The listing builds one solid part. Answer for the finished solid, in the listing's coordinates (mm). Face numbers are marked on the shaded views. A direction names the side the tool comes from. Round coordinates to 2 decimals unless told otherwise and drop trailing zeros. Order: outer loops, then holes, each group sorted by start corner. A loop starts at its lowest first (then second) coordinate and runs counter-clockwise, first axis right, second up. Notation, with made-up numbers: (-34.5, 68.5) -> (-0.5, 68.5) arc R19 ccw to (-0.5, 103.5) -> close; hole circle Ø9 at (38.5, 34). An arc over 180 degrees is marked (long way). Return JSON: item names as keys, results as strings. Group by question number.
(1) Determine the mould class of the marked faces 3, 4 and 5 for opening direction Z: +Z half, -Z half, draft (parallel to the pull), parting line (faces both ways), or undercut.
(2) The part is cut by section B-B (z = 0). Determine the outline of the cut face in (x, y), plus the area to 3 significant figures.
(3) Which of the six approach directions +Z, -Z, +X, -X, +Y, -Y give full straight-line access (tool end or side, diameter ignored) to the marked faces 1 and 2?
(4) The part is cut by section C-C (z = 5). Determine the outline of the cut face in (x, y), plus the area to 3 significant figures.
(5) The part is cut by section A-A (y = 0). Determine the outline of the cut face in (x, z).
(6) Each of these flat-tipped pins is pushed along its axis until it touches: pin 1 (12 mm diameter, centred on x = 34, y = 11.5, fed in from +Z); pin 2 (4.5 mm diameter, centred on x = 53, y = -4.5, fed in from +Z); pin 3 (5 mm diameter, centred on x = 73.5, z = 12.5, fed in from +Y). Where does it stop, or does it pass through?
(7) The part is cut by section D-D (y = -9.5). Determine the outline of the cut face in (x, z), plus the area to 3 significant figures.
(8) Consider line 1 (X direction, y = -4, z = 2.5); line 2 (Z direction, x = 28, y = -0.5); line 3 (Y direction, x = 83.5, z = -7.5). Determine where each line is inside the solid, lowest interval first. Write a range as [from, to].
from build123d import *

# Parameters (mm, degrees)
SKETCH1_R                           = 20
BOSS_EXTRUDE1_DEPTH                 = 105
CUT_EXTRUDE1_REACH                  = 110.743
CUT_EXTRUDE1_END_RADIUS             = 20
SKETCH2_W                           = 15
SKETCH2_H                           = 15
CUT_EXTRUDE1_DIRECTION_2_REACH      = 110.743
CUT_EXTRUDE1_DIRECTION_2_END_RADIUS = 20


with BuildPart() as part:
    # Sketch1 → Boss-Extrude1 (new body)
    with BuildSketch(Plane(origin=(0, 0, 0), x_dir=(0, 0, -1), z_dir=(1, 0, 0))):
        Circle(SKETCH1_R)
    extrude(amount=BOSS_EXTRUDE1_DEPTH)

    # Cut-Extrude1: up to this cylinder (the profile starts inside it)
    cut_extrude1_end = Plane(origin=(52.5, 0, 0), z_dir=(-1, 0, 0)) * Cylinder(CUT_EXTRUDE1_END_RADIUS, 262.486, mode=Mode.PRIVATE)
    # Sketch2 → Cut-Extrude1 (cut, up to the surface)
    with BuildSketch(Plane(origin=(0, 0, 0), x_dir=(1, 0, 0), z_dir=(0, 1, 0)), mode=Mode.PRIVATE) as cut_extrude1_sk1:
        with Locations((52.5, 0)):
            Rectangle(SKETCH2_W, SKETCH2_H)
    cut_extrude1_tool1 = extrude(cut_extrude1_sk1.sketch, amount=-CUT_EXTRUDE1_REACH, mode=Mode.PRIVATE) & cut_extrude1_end
    add(cut_extrude1_tool1.solids().sort_by_distance((52.5, 0, 0))[0], mode=Mode.SUBTRACT)

    # Cut-Extrude1 direction 2: up to this cylinder (the profile starts inside it)
    cut_extrude1_direction_2_end = Plane(origin=(52.5, 0, 0), z_dir=(-1, 0, 0)) * Cylinder(CUT_EXTRUDE1_DIRECTION_2_END_RADIUS, 262.486, mode=Mode.PRIVATE)
    # Sketch2 → Cut-Extrude1 direction 2 (cut, up to the surface)
    with BuildSketch(Plane(origin=(0, 0, 0), x_dir=(1, 0, 0), z_dir=(0, 1, 0)), mode=Mode.PRIVATE) as cut_extrude1_direction_2_sk1:
        with Locations((52.5, 0)):
            Rectangle(SKETCH2_W, SKETCH2_H)
    cut_extrude1_direction_2_tool1 = extrude(cut_extrude1_direction_2_sk1.sketch, amount=CUT_EXTRUDE1_DIRECTION_2_REACH, mode=Mode.PRIVATE) & cut_extrude1_direction_2_end
    add(cut_extrude1_direction_2_tool1.solids().sort_by_distance((52.5, 0, 0))[0], mode=Mode.SUBTRACT)


solid = part.part
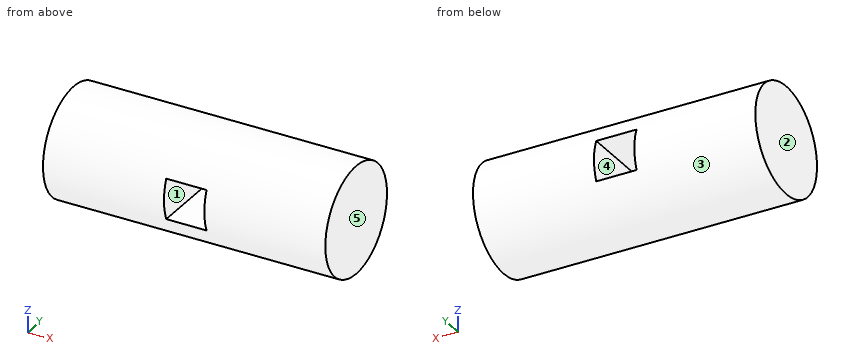
Answer below:
{
 "1": {"face 3": "parting line", "face 4": "undercut", "face 5": "draft"},
 "2": {"outline": "(0, -20) -> (45, -20) -> (45, 20) -> (0, 20) -> close; (60, -20) -> (105, -20) -> (105, 20) -> (60, 20) -> close", "area": "3,600 mm²"},
 "3": {"face 1": "+Y, -Y", "face 2": "+Z, -Z, -X, +Y, -Y"},
 "4": {"outline": "(0, -19.36) -> (45, -19.36) -> (45, 19.36) -> (0, 19.36) -> close; (60, -19.36) -> (105, -19.36) -> (105, 19.36) -> (60, 19.36) -> close", "area": "3,490 mm²"},
 "5": {"outline": "(0, -20) -> (105, -20) -> (105, 20) -> (0, 20) -> close; hole (45, -7.5) -> (60, -7.5) -> (60, 7.5) -> (45, 7.5) -> close"},
 "6": {"pin 1": "stops at z = 19.23", "pin 2": "stops at z = 19.87", "pin 3": "stops at y = 17.32"},
 "7": {"outline": "(0, -17.6) -> (105, -17.6) -> (105, 17.6) -> (0, 17.6) -> close; hole (45, -7.5) -> (60, -7.5) -> (60, 7.5) -> (45, 7.5) -> close", "area": "3,470 mm²"},
 "8": {"line 1": "x = [0, 45], [60, 105]", "line 2": "z = [-19.99, 19.99]", "line 3": "y = [-18.54, 18.54]"}
}
